```python
from build123d import *

# Parameters (mm, degrees)
SKETCH1_W           = 20
SKETCH1_H           = 20
BOSS_EXTRUDE1_DEPTH = 20
BOSS_EXTRUDE2_DEPTH = 20
BOSS_EXTRUDE3_DEPTH = 20
BOSS_EXTRUDE4_DEPTH = 20
BOSS_EXTRUDE5_DEPTH = 20


with BuildPart() as part:
    # Sketch1 → Boss-Extrude1 (new body)
    with BuildSketch(Plane.XY):
        Rectangle(SKETCH1_W, SKETCH1_H)
    extrude(amount=BOSS_EXTRUDE1_DEPTH)

    # Sketch2 → Boss-Extrude2 (add)
    with BuildSketch(Plane.XY.offset(20)):
        Polygon((2.85, 10), (2.85, 8), (4.8, 8), (4.8, 6), (2.5, 4), (-2.5, 4), (-4.8, 6), (-4.8, 8), (-2.85, 8), (-2.85, 10), align=None)
    extrude(amount=BOSS_EXTRUDE2_DEPTH)

    # Sketch3 → Boss-Extrude3 (add)
    with BuildSketch(Plane.XY.offset(20)):
        Polygon((-10, 2.85), (-8, 2.85), (-8, 4.8), (-6, 4.8), (-4, 2.5), (-4, -2.5), (-6, -4.8), (-8, -4.8), (-8, -2.85), (-10, -2.85), align=None)
    extrude(amount=BOSS_EXTRUDE3_DEPTH)

    # Sketch4 → Boss-Extrude4 (add)
    with BuildSketch(Plane.XY.offset(20)):
        Polygon((10, 2.85), (8, 2.85), (8, 4.8), (6, 4.8), (4, 2.5), (4, -2.689613267), (5.983673404, -4.989613267), (7.967346808, -4.989613267), (7.967346808, -2.85), (10, -2.85), align=None)
    extrude(amount=BOSS_EXTRUDE4_DEPTH)

    # Sketch5 → Boss-Extrude5 (add)
    with BuildSketch(Plane.XZ.offset(10)):
        Polygon((-10, 12.85), (-8, 12.85), (-8, 14.8), (-6, 14.8), (-4, 12.5), (-4, 7.5), (-6, 5.2), (-8, 5.2), (-8, 7.15), (-10, 7.15), align=None)
        Polygon((10, 12.85), (8, 12.85), (8, 14.8), (6, 14.8), (4, 12.5), (4, 7.5), (6, 5.2), (8, 5.2), (8, 7.15), (10, 7.15), align=None)
        Polygon((-2.85, 0), (2.85, 0), (2.85, 2), (4.8, 2), (4.8, 4), (2.5, 6), (-2.5, 6), (-4.8, 4), (-4.8, 2), (-2.85, 2), align=None)
    extrude(amount=BOSS_EXTRUDE5_DEPTH)


solid = part.part
```
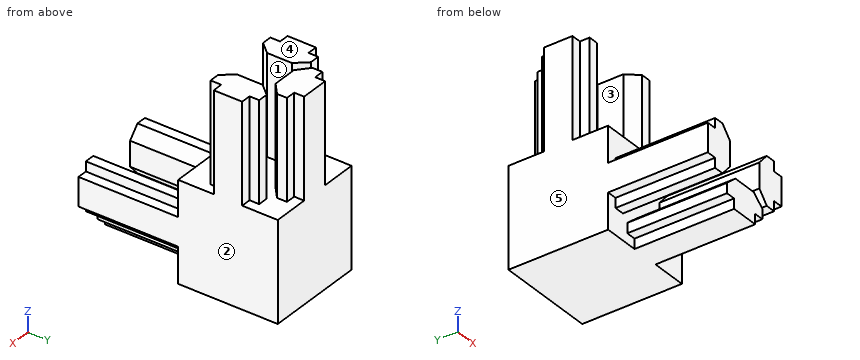
CAD build for the part. Positions are in the model's coordinates, mm. Face numbers are marked on the shaded views. A direction names the side the tool comes from. Give positions to 0.01 mm unless a question says otherwise; leave off trailing zeros. Order: outer loops, then holes, each group sorted by start corner. A loop starts at its lowest first (then second) coordinate and runs counter-clockwise, first axis right, second up. Notation, with made-up numbers: M 50,-33.75 L 103,-33.75 A31 ccw 103,5.25 Z; hole C 74,6.5 d2. An arc over 180 degrees is marked long. Put each result on its own line as item: value. Start each with the question number.
(1) Saw through at D-D, the plane y = -0.5. Write the cut outline in (x, z).
(2) Saw through at C-C, the plane x = 8.5. Write the cut outline in (y, z).
(3) Drill centre lines: line 1 along X through (y, z) = (1, 26); line 2 along Y through (x, z) = (1.75, 21); line 3 along Z through (x, y) = (4, 4). Where is each one in solid material? Low to high.
(4) Flat gauge pins, fed straight in: pin 1 Ø1.5 at (x, z) = (-1, 26) entering from -Y; pin 2 Ø2.5 at (x, y) = (0, -21.5) entering from +Z; pin 3 Ø12 at (x, y) = (4, -12.5) entering from +Z. Where does each tip first touch, or does it go through?
(5) Saw through at A-A, the plane z = 32. Give the number of separate pieces and of enclosed holes in the cut face, then the cut area to 3 significant figures.
(6) Which spindle directions (+Z, -Z, +X, -X, +Y, -Y) get a long thin tool onto all of the face, cutting with end or side? Do the marked faces 1 and 2. Say none if no direction does.
(7) Mould opens along X. For the marked faces 3, 4 and 5 say: +X half, -X half, draft (parallel to the pull), parting line (faces both ways), or undercut.
Check result:
1. outline: M -10,0 L 10,0 L 10,40 L 4,40 L 4,20 L -4,20 L -4,40 L -10,40 Z
2. outline: M -30,7.15 L -10,7.15 L -10,0 L 10,0 L 10,20 L 2.85,20 L 2.85,40 L -2.85,40 L -2.85,20 L -10,20 L -10,12.85 L -30,12.85 Z
3. line 1: x = -10 to -4, 4 to 10
3. line 2: y = 4 to 10
3. line 3: z = 0 to 20
4. pin 1: stops at y = 4
4. pin 2: stops at z = 6
4. pin 3: stops at z = 20
5. separate pieces: 3
5. enclosed holes: 0
5. area: 136 mm2
6. face 1: +Z, -Y
6. face 2: +Z, -Z, +X, +Y, -Y
7. face 3: undercut
7. face 4: draft
7. face 5: -X half
